```python
from build123d import *

# Parameters (mm, degrees)
MODEL_R             = 1.350108094
MODEL_R_2           = 1.30010409
MODEL_W             = 12.000960833
MODEL_H             = 22.8
BOSS_EXTRUDE1_DEPTH = 3


with BuildPart() as part:
    # Model → Boss-Extrude1 (new body)
    with BuildSketch(Plane.XY):
        with BuildLine():
            Line((58.668697195, 41.004775949), (61.668697195, 41.004775949))
            Line((61.668697195, 41.004775949), (61.668697195, 24.003921827))
            ThreePointArc((61.668697195, 24.003921827), (60.754304786, 21.847009523), (58.568180571, 21.004842626))
            Line((58.568180571, 21.004842626), (40.767051953, 21.004842626))
            ThreePointArc((40.767051953, 21.004842626), (38.710492919, 21.917586858), (37.866775535, 24.003414768))
            Line((37.866775535, 24.003414768), (37.866775535, 41.004775949))
            Line((37.866775535, 41.004775949), (40.867015743, 41.004775949))
            Line((40.867015743, 41.004775949), (40.867015743, 53.004775949))
            Line((40.867015743, 53.004775949), (37.866775535, 53.004775949))
            Line((37.866775535, 53.004775949), (37.866775535, 60.663449882))
            ThreePointArc((37.866775535, 60.663449882), (38.797636626, 62.682660658), (40.862794137, 63.506577512))
            Line((40.862794137, 63.506577512), (58.472438386, 63.506577512))
            ThreePointArc((58.472438386, 63.506577512), (60.66612789, 62.754918404), (61.668697195, 60.663956941))
            Line((61.668697195, 60.663956941), (61.668697195, 53.004775949))
            Line((61.668697195, 53.004775949), (58.668697195, 53.004775949))
            Line((58.668697195, 53.004775949), (58.668697195, 41.004775949))
        make_face()
        with Locations((41.167245975, 60.70691038)):
            Circle(MODEL_R, mode=Mode.SUBTRACT)
        with Locations((58.168607156, 60.70691038)):
            Circle(MODEL_R, mode=Mode.SUBTRACT)
        with Locations((41.167245975, 33.504732491)):
            Circle(MODEL_R, mode=Mode.SUBTRACT)
        with Locations((58.168607156, 33.504732491)):
            Circle(MODEL_R, mode=Mode.SUBTRACT)
        with Locations((40.617301942, 24.003971828)):
            Circle(MODEL_R_2, mode=Mode.SUBTRACT)
        with Locations((58.718751199, 24.003971828)):
            Circle(MODEL_R_2, mode=Mode.SUBTRACT)
        with Locations((49.667616262, 46.904842626)):
            Rectangle(MODEL_W, MODEL_H, mode=Mode.SUBTRACT)
    extrude(amount=BOSS_EXTRUDE1_DEPTH)


solid = part.part
```
Geometry check sheet. Reference: the model listing, model coordinates, mm. A direction names the side the tool comes from. Round coordinates to 2 decimals unless told otherwise and drop trailing zeros. Order: outer loops, then holes, each group sorted by start corner. A loop starts at its lowest first (then second) coordinate and runs counter-clockwise, first axis right, second up. Notation, with made-up numbers: (40.25, -29) - (82.25, -29) arc R13 ccw to (82.25, -4) - close; hole circle Ø4 at (53, 2.5). An arc over 180 degrees is marked (long way). Use a Markdown table: item, result. Add a question column.
1) Section check C-C (z = 1). Record the cut outline in (x, y).
2) Section check A-A (y = 42). Record the cut outline in (x, z), then the cut area to 3 significant figures.
3) Section check B-B (x = 49.25). Record the cut outline in (y, z).
4) Thickness scan on line 1 along X through (y, z) = (24, 1.9); line 2 along X through (y, z) = (56, 0.7); line 3 along X through (y, z) = (50, 2.05). Record the ranges inside material, lowest first.
5) Mould release check, pull along X, two halves, no side actions. Record for faces 1 (the flat face through (50, 35.505, 1)), 2 (the cylindrical face through (38.733, 21.894, 1.479)), 3 (the flat face through (55.668, 47, 1)), 4 (the flat face through (50, 33, 3)): released by +X, released by -X, zero draft, split by the parting line, or undercut.
6) Gauge pin test, flat ends, axial feed: P1, Ø1.5, axis at y = 50, z = 1, coming from the +X side; P2, Ø1.6, axis at x = 41.17, y = 33.5, coming from the +Z side; P3, Ø8, axis at x = 44, y = 36.5, coming from the -Z side; P4, Ø0.9, axis at y = 48, z = 2, coming from the -X side. Record the tip position at first contact, or that the pin passes through.
7) Set-up check for faces 5 (the flat face through (43.667, 47, 1)), 6 (the flat face through (50, 33, 0)), 7 (the flat face through (58.669, 47, 1)), 8 (the flat face through (40.867, 47, 1)): record each of +Z, -Z, +X, -X, +Y, -Y from which the full face is reachable in a straight line by a thin tool's end or side.
Established:
| question | item | result |
|---|---|---|
| 1 | outline | (37.87, 24) arc R3 ccw to (40.77, 21) - (58.57, 21) arc R3 ccw to (61.67, 24) - (61.67, 41) - (58.67, 41) - (58.67, 53) - (61.67, 53) - (61.67, 60.66) arc R3 ccw to (58.47, 63.51) - (40.86, 63.51) arc R3 ccw to (37.87, 60.66) - (37.87, 53) - (40.87, 53) - (40.87, 41) - (37.87, 41) - close; hole circle Ø2.6 at (40.62, 24); hole circle Ø2.7 at (41.17, 33.5); hole circle Ø2.7 at (41.17, 60.71); hole (43.67, 35.5) - (55.67, 35.5) - (55.67, 58.3) - (43.67, 58.3) - close; hole circle Ø2.7 at (58.17, 33.5); hole circle Ø2.7 at (58.17, 60.71); hole circle Ø2.6 at (58.72, 24) |
| 2 | outline | (40.87, 0) - (43.67, 0) - (43.67, 3) - (40.87, 3) - close; (55.67, 0) - (58.67, 0) - (58.67, 3) - (55.67, 3) - close |
| 2 | area | 17.4 mm2 |
| 3 | outline | (21, 0) - (35.5, 0) - (35.5, 3) - (21, 3) - close; (58.3, 0) - (63.51, 0) - (63.51, 3) - (58.3, 3) - close |
| 4 | line 1 | 37.87 to 39.32, 41.92 to 57.42, 60.02 to 61.67 |
| 4 | line 2 | 37.87 to 43.67, 55.67 to 61.67 |
| 4 | line 3 | 40.87 to 43.67, 55.67 to 58.67 |
| 5 | face 1 | undercut |
| 5 | face 2 | released by -X |
| 5 | face 3 | undercut |
| 5 | face 4 | zero draft |
| 6 | P1 | x = 58.67 |
| 6 | P2 | through |
| 6 | P3 | z = 0 |
| 6 | P4 | x = 40.87 |
| 7 | face 5 | +Z, -Z |
| 7 | face 6 | -Z, +X, -X, +Y, -Y |
| 7 | face 7 | +Z, -Z, +X |
| 7 | face 8 | +Z, -Z, -X |
